CAD build for the part. Positions are in the model's coordinates, mm. A direction names the side the tool comes from. Give positions to 0.01 mm unless a question says otherwise; leave off trailing zeros. Write each loop counter-clockwise with the first axis right and the second up, starting at its lowest first coordinate (ties: lowest second). Pieces come first, ordered by that corner, then holes. Notation, with made-up numbers: M 59.25,82.5 L 75.25,82.5 A21 ccw 75.25,93.5 Z; hole C -11,81 d10. An arc over 180 degrees is marked long. One line per question, with ' | ' between items. Start each with the question number.
1. Cut at D-D, the plane x = -9.5. Write the cut outline in (y, z), then the cut area to 3 significant figures.
2. Flat gauge pins, fed straight in: pin 1 (3 mm diameter, centred on y = 10, z = 7, fed in from +X); pin 2 (6 mm diameter, centred on x = 18, z = -2.5, fed in from +Y); pin 3 (1.4 mm diameter, centred on x = -30, y = 5.5, fed in from +Z). Where does each tip first touch, or does it go through?
3. Cut at B-B, the plane z = -10.25. Write the cut outline in (x, y), then the cut area to 3 significant figures.
4. Wall check: L1, parallel to X at y = 5.75, z = 2.75; L2, parallel to Z at x = 21, y = 11; L3, parallel to X at y = 19.75, z = -9. Give the ranges that are in metal, low to high.
5. Cut at C-C, the plane z = 5.75. Write the cut outline in (x, y).
6. Which spindle directions (+Z, -Z, +X, -X, +Y, -Y) get a long thin tool onto all of the face, cutting with end or side? Do faces 1 (the face through (24.25, 12, -1)), 2 (the face through (30, 7, -7.75)), 3 (the face through (0, 0, 1)). Say none if no direction does.
7. Pull direction Y, two halves, no side cores. Call faces 4 (the face through (32.52, 1.2, -10.28)), 5 (the face through (-24.25, 12, -1)), 6 (the face through (-29.535, 2.975, -10.285)), 7 (the face through (-29.498, 12.969, -10.077)): released by +Y, released by -Y, zero draft, split by the parting line, or undercut.
8. Cut at A-A, the plane y = 2.75. Write the cut outline in (x, z).
```python
from build123d import *

# Parameters (mm, degrees)
SKETCH1_W           = 52.5
SKETCH1_H           = 27.5
BOSS_EXTRUDE1_DEPTH = 2
BOSS_EXTRUDE2_DEPTH = 20
FILLET1_R           = 2
SKETCH3_R           = 0.75
BOSS_EXTRUDE3_DEPTH = 5
FILLET3_R           = 2


with BuildPart() as part:
    # Sketch1 → Boss-Extrude1 (new body)
    with BuildSketch(Plane(origin=(0, 0, 0), x_dir=(1, 0, 0), z_dir=(0, 1, 0))):
        with Locations((0, -1)):
            Rectangle(SKETCH1_W, SKETCH1_H)
    extrude(amount=BOSS_EXTRUDE1_DEPTH)

    # Sketch2 → Boss-Extrude2 (add)
    with BuildSketch(Plane(origin=(0, 2, 0), x_dir=(1, 0, 0), z_dir=(0, 1, 0))):
        Polygon((26.25, -14.75), (26.25, 12.75), (24.25, 12.75), (24.25, -12.75), (-24.25, -12.75), (-24.25, 12.75), (-26.25, 12.75), (-26.25, -14.75), align=None)
    extrude(amount=BOSS_EXTRUDE2_DEPTH)

    # Fillet1
    fillet1_edges = [part.edges().sort_by_distance(p)[0] for p in [
        (24.25, 12, 12.75),
        (-24.25, 12, 12.75),
        (26.25, 11, 14.75),
        (-26.25, 11, 14.75),
    ]]
    fillet(fillet1_edges, radius=FILLET1_R)

    # Sketch3 → Boss-Extrude3 (add)
    with BuildSketch(Plane(origin=(0, 0, -12.75), x_dir=(-1, 0, 0), z_dir=(0, 0, -1))):
        with BuildLine():
            Line((-26.25, 22), (-32.837765597, 3.680574669))
            ThreePointArc((-32.837765597, 3.680574669), (-32.499620006, 1.168320567), (-30.25, 0))
            Line((-30.25, 0), (-26.25, 0))
            Line((-26.25, 0), (-26.25, 22))
        make_face()
        with Locations((-30.25, 2.75)):
            Circle(SKETCH3_R, mode=Mode.SUBTRACT)
    boss_extrude3 = extrude(amount=-BOSS_EXTRUDE3_DEPTH)

    # Mirror3: Boss-Extrude3 across plane
    add(boss_extrude3.mirror(Plane(origin=(0, 0, 0), x_dir=(0, 0, 1), z_dir=(1, 0, 0))))

    # Fillet3
    fillet3_edges = [part.edges().sort_by_distance(p)[0] for p in [
        (26.25, 11, -7.75),
        (-26.25, 11, -7.75),
    ]]
    fillet(fillet3_edges, radius=FILLET3_R)


solid = part.part
```
Here are the results:
1) outline: M 0,-12.75 L 2,-12.75 L 2,12.75 L 22,12.75 L 22,14.75 L 0,14.75 Z | area: 95.0 mm^2
2) pin 1: x = 26.25 | pin 2: y = 2 | pin 3: z = -7.75
3) outline: M -32.84,3.68 A2.75 ccw -30.25,0 L 30.25,0 A2.75 ccw 32.84,3.68 L 26.25,22 L 24.25,22 L 24.25,2 L -24.25,2 L -24.25,22 L -26.25,22 Z; hole C -30.25,2.75 d1.5; hole C 30.25,2.75 d1.5 | area: 348 mm^2
4) L1: -26.25 to -24.25, 24.25 to 26.25 | L2: 12.75 to 14.75 | L3: -27.06 to -24.25, 24.25 to 27.06
5) outline: M -26.25,0 L 26.25,0 L 26.25,22 L 24.25,22 L 24.25,2 L -24.25,2 L -24.25,22 L -26.25,22 Z
6) face 1: -Z, +Y | face 2: +Z, +X, +Y, -Y | face 3: +Z, -Z, +X, -X, -Y
7) face 4: split by the parting line | face 5: zero draft | face 6: undercut | face 7: released by +Y
8) outline: M -33,-12.75 L -31,-12.75 L -31,-7.75 L -33,-7.75 Z; M -29.5,-12.75 L -24.25,-12.75 L -24.25,10.75 A2 cw -22.25,12.75 L 22.25,12.75 A2 cw 24.25,10.75 L 24.25,-12.75 L 29.5,-12.75 L 29.5,-7.75 L 28.25,-7.75 A2 cw 26.25,-5.75 L 26.25,12.75 A2 ccw 24.25,14.75 L -24.25,14.75 A2 ccw -26.25,12.75 L -26.25,-5.75 A2 cw -28.25,-7.75 L -29.5,-7.75 Z; M 31,-12.75 L 33,-12.75 L 33,-7.75 L 31,-7.75 Z
